from build123d import *

# Parameters (mm, degrees)
SKETCH1_W                      = 50
SKETCH1_H                      = 11
SKETCH1_R                      = 2.5
BASE_FLANGE1_DEPTH             = 1.5
EDGE_FLANGE1_STRIP_W           = 7.4732
EDGE_FLANGE1_STRIP_H           = 1.5
EDGE_FLANGE1_STRIP_CUT_DEPTH   = 50
EDGE_FLANGE1_STRIP_2_W         = 7.4732
EDGE_FLANGE1_STRIP_2_H         = 1.5
EDGE_FLANGE1_STRIP_CUT_2_DEPTH = 50
EDGE_FLANGE1_DEPTH             = 50
EDGE_FLANGE1_BEND_DEPTH        = 50
SKETCH10_R                     = 3
TAB2_DEPTH                     = 1.5


# Sheet-metal steps are written as plain solids
with BuildPart() as part:
    # Sketch1 → Base-Flange1 (new body)
    with BuildSketch(Plane.XY):
        Rectangle(SKETCH1_W, SKETCH1_H)
        with Locations((-20, 0)):
            Circle(SKETCH1_R, mode=Mode.SUBTRACT)
        with Locations((20, 0)):
            Circle(SKETCH1_R, mode=Mode.SUBTRACT)
    extrude(amount=-BASE_FLANGE1_DEPTH)

    # Edge-Flange1 strip (across the edge) → Edge-Flange1 strip cut (cut)
    with BuildSketch(Plane(origin=(-25, 5.5, -1.5), x_dir=(0, -1, 0), z_dir=(1, 0, 0))):
        with Locations((-3, -0.75)):
            Rectangle(EDGE_FLANGE1_STRIP_W, EDGE_FLANGE1_STRIP_H)
    extrude(amount=EDGE_FLANGE1_STRIP_CUT_DEPTH, mode=Mode.SUBTRACT)

    # Edge-Flange1 strip 2 (across the edge) → Edge-Flange1 strip cut 2 (cut)
    with BuildSketch(Plane(origin=(25, -5.5, -1.5), x_dir=(0, 1, 0), z_dir=(-1, 0, 0))):
        with Locations((-3, -0.75)):
            Rectangle(EDGE_FLANGE1_STRIP_2_W, EDGE_FLANGE1_STRIP_2_H)
    extrude(amount=EDGE_FLANGE1_STRIP_CUT_2_DEPTH, mode=Mode.SUBTRACT)

    # Edge-Flange1 section (across the edge) → Edge-Flange1 (add)
    with BuildSketch(Plane(origin=(-25, 5.5, -1.5), x_dir=(0, -1, 0), z_dir=(1, 0, 0))):
        with BuildLine():
            Line((-1.5, 0.7366), (-1.5, 5))
            Line((-1.5, 5), (0, 5))
            Line((0, 5), (0, 0.7366))
            ThreePointArc((0, 0.7366), (0.215745145, 0.215745145), (0.7366, 0))
            Line((0.7366, 0), (0.7366, -1.5))
            ThreePointArc((0.7366, -1.5), (-0.844915027, -0.844915027), (-1.5, 0.7366))
        make_face()
    extrude(amount=EDGE_FLANGE1_DEPTH)

    # Edge-Flange1 section 2 (across the edge) → Edge-Flange1 bend (add)
    with BuildSketch(Plane(origin=(25, -5.5, -1.5), x_dir=(0, 1, 0), z_dir=(-1, 0, 0))):
        with BuildLine():
            Line((-1.5, 0.7366), (-1.5, 5))
            Line((-1.5, 5), (0, 5))
            Line((0, 5), (0, 0.7366))
            ThreePointArc((0, 0.7366), (0.215745145, 0.215745145), (0.7366, 0))
            Line((0.7366, 0), (0.7366, -1.5))
            ThreePointArc((0.7366, -1.5), (-0.844915027, -0.844915027), (-1.5, 0.7366))
        make_face()
    extrude(amount=EDGE_FLANGE1_BEND_DEPTH)

    # Sketch10 → Tab2 (add)
    with BuildSketch(Plane(origin=(0, 7, 0), x_dir=(1, 0, 0), z_dir=(0, 1, 0))):
        with BuildLine():
            Line((-15, 6.5), (-4.269254688, 24.102588021))
            ThreePointArc((-4.269254688, 24.102588021), (0, 26.5), (4.269254688, 24.102588021))
            Line((4.269254688, 24.102588021), (15, 6.5))
            Line((15, 6.5), (-15, 6.5))
        make_face()
        with Locations(Location((0, 21.5, 0), (0, 0, 270))):
            Circle(SKETCH10_R, mode=Mode.SUBTRACT)
    tab2 = extrude(amount=-TAB2_DEPTH)

    # Mirror1: Tab2 across plane
    add(tab2.mirror(Plane.ZX))


solid = part.part
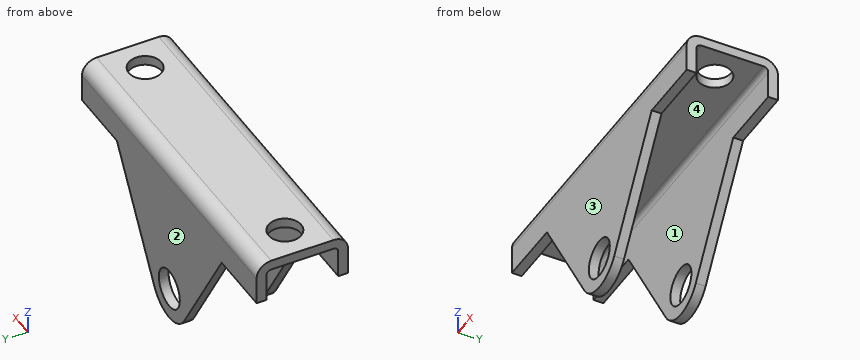
Here's how the part is built. I have some questions about the finished solid (model axes, mm). Face numbers are marked on the shaded views. Round coordinates to 2 decimals unless told otherwise and drop trailing zeros. Write each loop counter-clockwise with the first axis right and the second up, starting at its lowest first coordinate (ties: lowest second). Pieces come first, ordered by that corner, then holes.
1. If we mould it in two halves opening along Y, with no side actions, what happens to the marked faces 1, 2, 3 and 4? For each: released by +Y, released by -Y, zero draft, split by the parting line, or undercut.
2. Suppose I cut it at C-C (z = -22). List the corners of the cut face in (x, y) for me.
3. Suppose I cut it at A-A (y = 0). List the corners of the cut face in (x, z) for me, and give its area (3 significant figures).
4. Suppose I cut it at B-B (x = 0). List the corners of the cut face in (y, z) for me.
5. I need wall thicknesses on L1, parallel to Y at x = 3, z = -6; L2, parallel to Z at x = -14, y = -2.5; L3, parallel to X at y = 5.9, z = -21.5. Which ranges of each line are inside material? Lowest first, please.
6. Will these pins go through, and if not, where does the flat tip stop? pin 1 Ø3 at (x, y) = (-20, 0) entering from -Z; pin 2 Ø1.6 at (x, y) = (18, 6.5) entering from -Z; pin 3 Ø9.5 at (x, z) = (0, -21.5) entering from -Y; pin 4 Ø8 at (x, y) = (20, 0) entering from -Z.
7. Suppose I cut it at D-D (x = 20). List the corners of the cut face in (y, z) for me.
Answer sheet:
1. face 1: undercut
1. face 2: released by +Y
1. face 3: released by -Y
1. face 4: undercut
2. outline: (-5.55, -7) - (-2.96, -7) - (-2.96, -5.5) - (-5.55, -5.5) - close; (-5.55, 5.5) - (-2.96, 5.5) - (-2.96, 7) - (-5.55, 7) - close; (2.96, -7) - (5.55, -7) - (5.55, -5.5) - (2.96, -5.5) - close; (2.96, 5.5) - (5.55, 5.5) - (5.55, 7) - (2.96, 7) - close
3. outline: (-25, -1.5) - (-22.5, -1.5) - (-22.5, 0) - (-25, 0) - close; (-17.5, -1.5) - (17.5, -1.5) - (17.5, 0) - (-17.5, 0) - close; (22.5, -1.5) - (25, -1.5) - (25, 0) - (22.5, 0) - close
3. area: 60.0 mm2
4. outline: (-7, -26.5) - (-5.5, -26.5) - (-5.5, -24.5) - (-7, -24.5) - close; (-7, -18.5) - (-5.5, -18.5) - (-5.5, -2.24) arc R0.74 cw to (-4.76, -1.5) - (4.76, -1.5) arc R0.74 cw to (5.5, -2.24) - (5.5, -18.5) - (7, -18.5) - (7, -2.24) arc R2.24 ccw to (4.76, 0) - (-4.76, 0) arc R2.24 ccw to (-7, -2.24) - close; (5.5, -26.5) - (7, -26.5) - (7, -24.5) - (5.5, -24.5) - close
5. L1: y = -7 to -5.5, 5.5 to 7
5. L2: z = -1.5 to 0
5. L3: x = -5.86 to -3, 3 to 5.86
6. pin 1: passes through
6. pin 2: stops at z = -6.5
6. pin 3: stops at y = -7
6. pin 4: stops at z = -1.5
7. outline: (-7, -6.5) - (-5.5, -6.5) - (-5.5, -2.24) arc R0.74 cw to (-4.76, -1.5) - (-2.5, -1.5) - (-2.5, 0) - (-4.76, 0) arc R2.24 ccw to (-7, -2.24) - close; (2.5, -1.5) - (4.76, -1.5) arc R0.74 cw to (5.5, -2.24) - (5.5, -6.5) - (7, -6.5) - (7, -2.24) arc R2.24 ccw to (4.76, 0) - (2.5, 0) - close
